The listing builds one solid part. Answer for the finished solid, in the listing's coordinates (mm). Face numbers are marked on the shaded views. A direction names the side the tool comes from. Round coordinates to 2 decimals unless told otherwise and drop trailing zeros. Write each loop counter-clockwise with the first axis right and the second up, starting at its lowest first coordinate (ties: lowest second). Pieces come first, ordered by that corner, then holes.
Item 1: Find the intervals of material crossed by probe 1 along Z at (x, y) = (-23, -9); probe 2 along Z at (x, y) = (4.5, -31.75); probe 3 along Z at (x, y) = (21, -41.5), in increasing order.
Item 2: Find section A-A on z = -24.5. Give the vertices of the cut face in (x, y).
Item 3: A tool of negligible diameter and unlimited length cuts with its end or side. For the marked faces 5, 6 and 7, from which of +Z, -Z, +X, -X, +Y, -Y can it reach the whole face along a straight path? Write none if from no direction.
Item 4: Each of these flat-tipped pins is pushed along its axis until it touches: pin 1 (1.9 mm diameter, centred on y = -11, z = 1, fed in from +X); pin 2 (6 mm diameter, centred on x = 3, y = -57, fed in from +Z) (3 decimals); pin 3 (7.5 mm diameter, centred on y = -53.5, z = 5.5, fed in from -X); pin 4 (8 mm diameter, centred on x = 23.5, z = -24.5, fed in from +Y). Where does it stop, or does it pass through?
Item 5: Find section B-B on z = 23.5. Give the vertices of the cut face in (x, y), then the cut area to 3 significant figures.
Item 6: For a pull along X with two mould halves and no side action, classify the marked faces 1, 2, 3 and 4 as +X half, -X half, draft (parallel to the pull), parting line (faces both ways), or undercut.
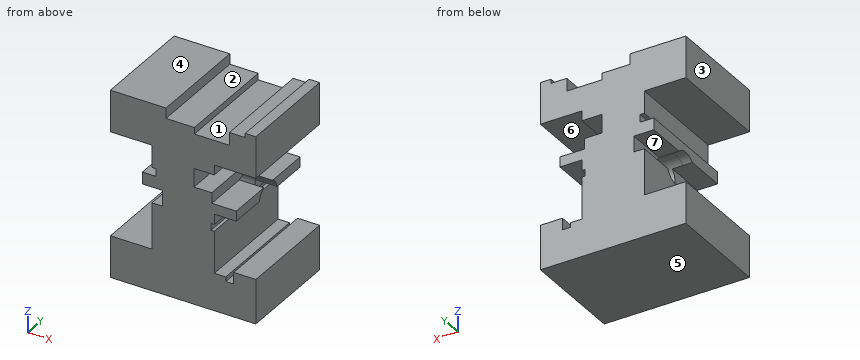
```python
from build123d import *

# Parameters (mm, degrees)
F1_DEPTH  = 63.5
F2_R      = 9.0561828793
F3_DEPTH  = 63.501
F4_W      = 17.3674514517
F4_H      = 63.5
F5_DEPTH  = 6.35
F6_W      = 9.6430126578
F6_H      = 63.5
F7_DEPTH  = 2.54
F8_DEPTH  = 10.3378
F9_W      = 63.5
F9_H      = 4.6800179407
F10_DEPTH = 2.54
F11_DEPTH = 6.35
F12_DEPTH = 6.35
F13_DEPTH = 5.842
F14_W     = 63.5
F14_H     = 11.3577079028
F15_DEPTH = 12.3698
F16_DEPTH = 13.462
F17_DEPTH = 13.462
F18_DEPTH = 1.524
F19_DEPTH = 1.9558
F20_DEPTH = 1.9558
F21_W     = 4.8483535647
F21_H     = 63.5
F22_DEPTH = 5.334
F23_DEPTH = 1.778
F24_DEPTH = 2.54


with BuildPart() as f1:
    # F0 (on Front) → F1 (new body)
    with BuildSketch(Plane.XZ):
        Polygon((-43.0088681884, -29.9449780501), (-43.0088681884, -55.3449780501), (45.8911318116, -55.3449780501), (45.8911318116, -29.9449780501), (20.4911318116, -29.9449780501), (20.4911318116, 33.5550219499), (45.8911318116, 33.5550219499), (45.8911318116, 58.9550219499), (-43.0088681884, 58.9550219499), (-43.0088681884, 33.5550219499), (-17.6088681884, 33.5550219499), (-17.6088681884, -29.9449780501), align=None)
    extrude(amount=F1_DEPTH)

    # F2 (on face) → F3 (cut, through all)
    with BuildSketch(Plane.YZ.offset(20.4911318116)):
        with Locations((-31.75, 1.8050219499)):
            Circle(F2_R)
    extrude(amount=-F3_DEPTH, mode=Mode.SUBTRACT)

    # F4 (on face) → F5 (cut)
    with BuildSketch(Plane.XY.offset(58.9550219499)):
        with Locations((-0.3427523188, -31.75)):
            Rectangle(F4_W, F4_H)
    extrude(amount=-F5_DEPTH, mode=Mode.SUBTRACT)

    # F6 (on face) → F7 (cut)
    with BuildSketch(Plane.XY.offset(58.9550219499)):
        with Locations((34.5854004845, -31.75)):
            Rectangle(F6_W, F6_H)
    extrude(amount=-F7_DEPTH, mode=Mode.SUBTRACT)

    # F8 (cut): a face of the model
    f8_faces = [f1.faces().sort_by_distance(p)[0] for p in [
        (19.0524337813, -31.75, 58.9550219499),
    ]]
    extrude(f8_faces, amount=-F8_DEPTH, mode=Mode.SUBTRACT)

    # F9 (on face) → F10 (cut)
    with BuildSketch(Plane(origin=(-17.6088681884, 0, 0), x_dir=(0, -1, 0), z_dir=(-1, 0, 0))):
        with Locations((31.75, 17.5831750967)):
            Rectangle(F9_W, F9_H)
    extrude(amount=-F10_DEPTH, mode=Mode.SUBTRACT)

    # F9 (on face) → F11 (cut)
    with BuildSketch(Plane(origin=(-17.6088681884, 0, 0), x_dir=(0, -1, 0), z_dir=(-1, 0, 0))):
        with BuildLine():
            Line((63.5, -1.6929475823), (63.5, 7.987478748))
            Line((63.5, 7.987478748), (38.3675279587, 7.987478748))
            ThreePointArc((38.3675279587, 7.987478748), (40.1744878701, 5.128040528), (40.8061828793, 1.8050219499))
            ThreePointArc((40.8061828793, 1.8050219499), (40.6287392884, 0.021083332), (40.1033620474, -1.6929475823))
            Line((40.1033620474, -1.6929475823), (63.5, -1.6929475823))
        make_face()
    extrude(amount=-F11_DEPTH, mode=Mode.SUBTRACT)

    # F9 (on face) → F12 (cut)
    with BuildSketch(Plane(origin=(-17.6088681884, 0, 0), x_dir=(0, -1, 0), z_dir=(-1, 0, 0))):
        with BuildLine():
            Line((25.1324720413, 7.987478748), (0, 7.987478748))
            Line((0, 7.987478748), (0, -1.6929475823))
            Line((0, -1.6929475823), (23.3966379526, -1.6929475823))
            ThreePointArc((23.3966379526, -1.6929475823), (22.8359913407, 3.4034267691), (25.1324720413, 7.987478748))
        make_face()
    extrude(amount=-F12_DEPTH, mode=Mode.SUBTRACT)

    # F9 (on face) → F13 (join)
    with BuildSketch(Plane(origin=(-17.6088681884, 0, 0), x_dir=(0, -1, 0), z_dir=(-1, 0, 0))):
        with BuildLine():
            Line((63.5, 7.987478748), (63.5, 15.2431661263))
            Line((63.5, 15.2431661263), (0, 15.2431661263))
            Line((0, 15.2431661263), (0, 7.987478748))
            Line((0, 7.987478748), (25.1324720413, 7.987478748))
            ThreePointArc((25.1324720413, 7.987478748), (31.75, 10.8612048292), (38.3675279587, 7.987478748))
            Line((38.3675279587, 7.987478748), (63.5, 7.987478748))
        make_face()
    extrude(amount=F13_DEPTH)

    # F14 (on face) → F15 (cut)
    with BuildSketch(Plane.YZ.offset(20.4911318116)):
        with Locations((-31.75, 21.8542935327)):
            Rectangle(F14_W, F14_H)
    extrude(amount=-F15_DEPTH, mode=Mode.SUBTRACT)

    # F14 (on face) → F16 (join)
    with BuildSketch(Plane.YZ.offset(20.4911318116)):
        with BuildLine():
            Line((-36.1157784174, 9.7394045442), (-63.5, 9.7394045442))
            Line((-63.5, 9.7394045442), (-63.5, 3.6062416621))
            Line((-63.5, 3.6062416621), (-40.6252496242, 3.6062416621))
            ThreePointArc((-40.6252496242, 3.6062416621), (-39.0462406508, 7.1696580707), (-36.1157784174, 9.7394045442))
        make_face()
    extrude(amount=F16_DEPTH)

    # F14 (on face) → F17 (join)
    with BuildSketch(Plane.YZ.offset(20.4911318116)):
        with BuildLine():
            Line((0, 3.6062416621), (0, 9.7394045442))
            Line((0, 9.7394045442), (-27.3842215826, 9.7394045442))
            ThreePointArc((-27.3842215826, 9.7394045442), (-24.4537593492, 7.1696580707), (-22.8747503758, 3.6062416621))
            Line((-22.8747503758, 3.6062416621), (0, 3.6062416621))
        make_face()
    extrude(amount=F17_DEPTH)

    # F14 (on face) → F18 (cut)
    with BuildSketch(Plane.YZ.offset(20.4911318116)):
        with BuildLine():
            Line((0, 16.1754395813), (-63.5, 16.1754395813))
            Line((-63.5, 16.1754395813), (-63.5, 9.7394045442))
            Line((-63.5, 9.7394045442), (-36.1157784174, 9.7394045442))
            ThreePointArc((-36.1157784174, 9.7394045442), (-31.75, 10.8612048292), (-27.3842215826, 9.7394045442))
            Line((-27.3842215826, 9.7394045442), (0, 9.7394045442))
            Line((0, 9.7394045442), (0, 16.1754395813))
        make_face()
    extrude(amount=-F18_DEPTH, mode=Mode.SUBTRACT)

    # F14 (on face) → F19 (cut)
    with BuildSketch(Plane.YZ.offset(20.4911318116)):
        with BuildLine():
            Line((-39.574901363, -2.7540752199), (-63.5, -2.7540752199))
            Line((-63.5, -2.7540752199), (-63.5, -6.8428497761))
            Line((-63.5, -6.8428497761), (-34.4386358909, -6.8428497761))
            ThreePointArc((-34.4386358909, -6.8428497761), (-37.3903134435, -5.2802665131), (-39.574901363, -2.7540752199))
        make_face()
    extrude(amount=-F19_DEPTH, mode=Mode.SUBTRACT)

    # F14 (on face) → F20 (cut)
    with BuildSketch(Plane.YZ.offset(20.4911318116)):
        with BuildLine():
            Line((0, -6.8428497761), (0, -2.7540752199))
            Line((0, -2.7540752199), (-23.925098637, -2.7540752199))
            ThreePointArc((-23.925098637, -2.7540752199), (-26.1096865565, -5.2802665131), (-29.0613641091, -6.8428497761))
            Line((-29.0613641091, -6.8428497761), (0, -6.8428497761))
        make_face()
    extrude(amount=-F20_DEPTH, mode=Mode.SUBTRACT)

    # F21 (on face) → F22 (cut)
    with BuildSketch(Plane.XY.offset(-29.9449780501)):
        with Locations((29.9499258399, -31.75)):
            Rectangle(F21_W, F21_H)
    extrude(amount=-F22_DEPTH, mode=Mode.SUBTRACT)

    # F23 (add): a face of the model
    f23_faces = [f1.faces().sort_by_distance(p)[0] for p in [
        (39.1326172169, -31.75, -29.9449780501),
    ]]
    extrude(f23_faces, amount=F23_DEPTH)

    # F24 (cut): a face of the model
    f24_faces = [f1.faces().sort_by_distance(p)[0] for p in [
        (24.0084404346, -31.75, -29.9449780501),
    ]]
    extrude(f24_faces, amount=-F24_DEPTH, mode=Mode.SUBTRACT)


solid = f1.part
```
Check values:
1. probe 1: z = -55.34 to -29.94, 7.99 to 15.24, 33.56 to 58.96
1. probe 2: z = -55.34 to -7.25, 10.86 to 52.61
1. probe 3: z = -55.34 to -32.48, 3.61 to 9.74, 33.56 to 48.62
2. outline: (-17.61, -63.5) - (20.49, -63.5) - (20.49, 0) - (-17.61, 0) - close
3. face 5: -Z, +X, -X, +Y, -Y
3. face 6: +X, +Y, -Y
3. face 7: -X, +Y, -Y
4. pin 1: stops at x = 20.49
4. pin 2: stops at z = 52.605
4. pin 3: stops at x = -23.45
4. pin 4: stops at y = 0
5. outline: (-17.61, -63.5) - (8.12, -63.5) - (8.12, 0) - (-17.61, 0) - close
5. area: 1,630 mm2
6. face 1: undercut
6. face 2: undercut
6. face 3: -X half
6. face 4: draft
